Build history of the part. All positions in model axes, mm. A direction names the side the tool comes from. Give positions to 0.01 mm unless a question says otherwise; leave off trailing zeros. Write each loop counter-clockwise with the first axis right and the second up, starting at its lowest first coordinate (ties: lowest second). Pieces come first, ordered by that corner, then holes. Notation, with made-up numbers: (73, 39.5) -> (96, 39.5) arc R28 ccw to (96, 65.5) -> close; hole circle Ø1 at (82, -18). An arc over 180 degrees is marked (long way). Write item = value, one per line. Start each with the question number.
Q1. Saw through at C-C, the plane z = 8.5. List the corners of the cut face in (x, y).
Q2. Saw through at B-B, the plane y = -2. List the corners of the cut face in (x, z).
Q3. Wall check: line 1 (Y direction, x = 4.35, z = 8.1); line 2 (Y direction, x = 4, z = 8); line 3 (Z direction, x = -4, y = -4). Give the ranges that are in metal, low to high.
Q4. Saw through at D-D, the plane z = 2.25. List the corners of the cut face in (x, y).
Q5. Drop flat-ended pins along their axis: P1, Ø1.9, axis at x = 1, y = 0, coming from the +Z side; P2, Ø10, axis at x = -9, y = 2.5, coming from the +Z side; P3, Ø6, axis at x = -4, z = 6.5, coming from the +Y side; P4, Ø5, axis at y = 5.5, z = 8.5, coming from the +X side. Give the stop position or say it passes through.
Q6. Mould opens along Y. For faces 3 (the face through (0, 0, 0)), 4 (the face through (4.316, 7.382, 6.553)), 5 (the face through (-2.63, -11.86, 4.93)) say: pulls with the +Y half, pulls with the -Y half, needs draft (parallel to the pull), parting line crosses it, or undercut.
Q7. Tool access for faces 1 (the face through (7.84, 0.27, 8.48)), 2 (the face through (0, 0, 16.5)): list every direction of +Z, -Z, +X, -X, +Y, -Y with a clear straight run to the whole face (end or side of a thin tool).
Q8. Saw through at A-A, the plane x = 0. List the corners of the cut face in (y, z), then the cut area to 3 significant figures.
from build123d import *

# Parameters (mm, degrees)
SKETCH1_R                  = 12.15
BOSS_EXTRUDE1_DEPTH        = 10
SKETCH2_R                  = 3.15
BOSS_EXTRUDE2_DEPTH        = 0.8
SKETCH3_R                  = 0.85
BOSS_EXTRUDE3_DEPTH        = 5.7
M1_6_CLEARANCE_HOLE1_D     = 1.8
M1_6_CLEARANCE_HOLE1_DEPTH = 3
M1_6_CLEARANCE_HOLE1_TIP   = 0.540774557


with BuildPart() as part:
    # Sketch1 → Boss-Extrude1 (new body)
    with BuildSketch(Plane.XY):
        Circle(SKETCH1_R)
    extrude(amount=BOSS_EXTRUDE1_DEPTH)

    # Sketch2 → Boss-Extrude2 (add)
    with BuildSketch(Plane.XY.offset(10)):
        Circle(SKETCH2_R)
    extrude(amount=BOSS_EXTRUDE2_DEPTH)

    # Sketch3 → Boss-Extrude3 (add)
    with BuildSketch(Plane.XY.offset(10.8)):
        Circle(SKETCH3_R)
    extrude(amount=BOSS_EXTRUDE3_DEPTH)

    # M1.6 Clearance Hole1
    with Locations(Plane.XY.offset(10)):
        with Locations((-4.35, 7.534421013), (4.35, 7.534421013), (8.7, 0), (4.35, -7.534421013), (-4.35, -7.534421013), (-8.7, 0)):
            Hole(M1_6_CLEARANCE_HOLE1_D / 2, depth=M1_6_CLEARANCE_HOLE1_DEPTH)
            with Locations((0, 0, -(M1_6_CLEARANCE_HOLE1_DEPTH + M1_6_CLEARANCE_HOLE1_TIP / 2))):  # 118° drill point
                Cone(0, M1_6_CLEARANCE_HOLE1_D / 2, M1_6_CLEARANCE_HOLE1_TIP, mode=Mode.SUBTRACT)


solid = part.part
Report:
q1.outline = circle Ø24.3 at (0, 0); hole circle Ø1.8 at (-8.7, 0); hole circle Ø1.8 at (-4.35, -7.53); hole circle Ø1.8 at (-4.35, 7.53); hole circle Ø1.8 at (4.35, -7.53); hole circle Ø1.8 at (4.35, 7.53); hole circle Ø1.8 at (8.7, 0)
q2.outline = (-11.98, 0) -> (11.98, 0) -> (11.98, 10) -> (2.43, 10) -> (2.43, 10.8) -> (-2.43, 10.8) -> (-2.43, 10) -> (-11.98, 10) -> close
q3.line_1 = -11.34 to -8.43, -6.63 to 6.63, 8.43 to 11.34
q3.line_2 = -11.47 to -8.36, -6.71 to 6.71, 8.36 to 11.47
q3.line_3 = 0 to 10
q4.outline = circle Ø24.3 at (0, 0)
q5.P1 = 16.5
q5.P2 = 10
q5.P3 = 12.11
q5.P4 = 11.77
q6.face_3 = needs draft
q6.face_4 = undercut
q6.face_5 = parting line crosses it
q7.face_1 = +Z
q7.face_2 = +Z, +X, -X, +Y, -Y
q8.outline = (-12.15, 0) -> (12.15, 0) -> (12.15, 10) -> (3.15, 10) -> (3.15, 10.8) -> (0.85, 10.8) -> (0.85, 16.5) -> (-0.85, 16.5) -> (-0.85, 10.8) -> (-3.15, 10.8) -> (-3.15, 10) -> (-12.15, 10) -> close
q8.area = 258 mm2
